Autodesk Inventor part; units mm, degrees
ref_plane "YZ Plane" through (0, 0, 0) normal (1, 0, 0) x (0, 1, 0)
ref_plane "XZ Plane" through (0, 0, 0) normal (0, 1, 0) x (-1, 0, 0)
ref_plane "XY Plane" through (0, 0, 0) normal (0, 0, 1) x (1, 0, 0)
ref_plane "Work Plane2" through (0, 5.2982, -18) normal (0, 0, -1) x (-1, 0, 0)
ref_plane "Work Plane4" through (0, -4.9464, -12) normal (0, 0, -1) x (-1, 0, 0)
ref_plane "Work Plane3" through (0, -4.9464, -7) normal (0, 0, -1) x (-1, 0, 0)
sketch "Sketch3" plane through (0, 5.2982, -18) normal (0, 0, -1) x (-1, 0, 0)
  line L0 (13, 53.6093) -> (-13, 53.6093)
  arc A0 (-13, 53.6093) -> (-30, 36.6093) centre (-13, 36.6093) ccw
  line L1 (-30, 36.6093) -> (-30, -44.3907)
  line L2 (-30, -44.3907) -> (30, -44.3907)
  line L3 (30, -44.3907) -> (30, 36.6093)
  arc A1 (30, 36.6093) -> (13, 53.6093) centre (13, 36.6093) ccw
  line L4 (-0.95, 23.6093) -> (-0.95, 40.6093)
  line L5 (-0.95, 40.6093) -> (0.95, 40.6093)
  line L6 (0.95, 40.6093) -> (0.95, 23.6093)
  line L7 (0.95, 23.6093) -> (-0.95, 23.6093)
  line L8 (6.55, 40.6093) -> (8.45, 40.6093)
  line L9 (8.45, 40.6093) -> (8.45, 23.6093)
  line L10 (8.45, 23.6093) -> (6.55, 23.6093)
  line L11 (6.55, 23.6093) -> (6.55, 40.6093)
  line L12 (-8.45, 40.6093) -> (-6.55, 40.6093)
  line L13 (-6.55, 40.6093) -> (-6.55, 23.6093)
  line L14 (-6.55, 23.6093) -> (-8.45, 23.6093)
  line L15 (-8.45, 23.6093) -> (-8.45, 40.6093)
  line L16 (-15.5, -21.0481) -> (-15.5, 10.5093)
  line L17 (-15.5, 10.5093) -> (-12, 10.5093)
  line L18 (-12, 10.5093) -> (-12, 4.9593)
  line L19 (-12, 4.9593) -> (12, 4.9593)
  line L20 (12, 4.9593) -> (12, 10.5093)
  line L21 (12, 10.5093) -> (15.5, 10.5093)
  line L22 (15.5, 10.5093) -> (15.5, -21.0481)
  arc A2 (17.5, -25.2907) -> (15.5, -21.0481) centre (12, -25.2907) ccw
  line L23 (17.5, -25.2907) -> (17.5, -34.7907)
  arc A3 (12, -40.2907) -> (17.5, -34.7907) centre (12, -34.7907) ccw
  line L24 (12, -40.2907) -> (-12, -40.2907)
  arc A4 (-17.5, -34.7907) -> (-12, -40.2907) centre (-12, -34.7907) ccw
  line L25 (-17.5, -34.7907) -> (-17.5, -25.2907)
  arc A5 (-15.5, -21.0481) -> (-17.5, -25.2907) centre (-12, -25.2907) ccw
  line L26 (-15.5, -0.3907) -> (15.5, -0.3907)
  line L27 (-15.5, -21.0481) -> (-15.5, -0.3907)
  arc A6 (-12, -19.7907) -> (-15.5, -21.0481) centre (-12, -25.2907) ccw
  line L28 (12, -19.7907) -> (-12, -19.7907)
  arc A7 (15.5, -21.0481) -> (12, -19.7907) centre (12, -25.2907) ccw
  line L29 (15.5, -0.3907) -> (15.5, -21.0481)
  arc A8 (-15, -21.2907) -> (-17, -25.2907) centre (-12, -25.2907) ccw
  line L30 (-17, -25.2907) -> (-17, -34.7907)
  arc A9 (-17, -34.7907) -> (-12, -39.7907) centre (-12, -34.7907) ccw
  line L31 (-12, -39.7907) -> (12, -39.7907)
  arc A10 (12, -39.7907) -> (17, -34.7907) centre (12, -34.7907) ccw
  line L32 (17, -34.7907) -> (17, -25.2907)
  arc A11 (17, -25.2907) -> (15, -21.2907) centre (12, -25.2907) ccw
  line L33 (-15, -21.2907) -> (-15, 10.0093)
  line L34 (-15, 10.0093) -> (-12.5, 10.0093)
  line L35 (-12.5, 10.0093) -> (-12.5, 4.4593)
  line L36 (-12.5, 4.4593) -> (12.5, 4.4593)
  line L37 (12.5, 4.4593) -> (12.5, 10.0093)
  line L38 (12.5, 10.0093) -> (15, 10.0093)
  line L39 (15, 10.0093) -> (15, -21.2907)
  point P0 (0, -5.2982)
  dimension "d3" = 0.5
  dimension "d4" = 0.5
extrude "Extrusion1" add sketch "Sketch3" against normal up to surface (5 mm away) from surface at -6 contours L33 L26 L39 A7 L28 A6 | A6 L28 A7 L39 A11 L32 A10 L31 A9 L30 A8 L33 | L33 L34 L35 L36 L37 L38 L39 L26
sketch "Sketch4" plane through (-12.5, 9.7575, -7) normal (0, 0, 1) x (1, 0, 0)
  line L0 (29.5, -39.25) -> (29.5, -29.75)
  arc A0 (29.5, -29.75) -> (27.5, -25.75) centre (24.5, -29.75) ccw
  line L1 (27.5, -25.75) -> (27.5, 5.55)
  line L2 (27.5, 5.55) -> (25, 5.55)
  line L3 (25, 5.55) -> (25, 0)
  line L4 (25, 0) -> (0, 0)
  line L5 (0, 0) -> (0, 5.55)
  line L6 (0, 5.55) -> (-2.5, 5.55)
  line L7 (-2.5, 5.55) -> (-2.5, -25.75)
  arc A1 (-2.5, -25.75) -> (-4.5, -29.75) centre (0.5, -29.75) ccw
  line L8 (-4.5, -29.75) -> (-4.5, -39.25)
  arc A2 (-4.5, -39.25) -> (0.5, -44.25) centre (0.5, -39.25) ccw
  line L9 (0.5, -44.25) -> (24.5, -44.25)
  arc A3 (24.5, -44.25) -> (29.5, -39.25) centre (24.5, -39.25) ccw
  line L10 (0.5, -24.25) -> (24.5, -24.25)
  arc A4 (0.5, -24.25) -> (-3, -25.5074) centre (0.5, -29.75) ccw
  arc A5 (28, -25.5074) -> (24.5, -24.25) centre (24.5, -29.75) ccw
  arc A6 (27.5, -25.75) -> (24.5, -24.75) centre (24.5, -29.75) ccw
  line L11 (24.5, -24.75) -> (0.5, -24.75)
  arc A7 (0.5, -24.75) -> (-2.5, -25.75) centre (0.5, -29.75) ccw
  point P0 (12.5, -9.7575)
extrude "Extrusion2" add sketch "Sketch4" along normal blind 6 contours A3 L9 A2 L8 A1 A7 L11 A6 A0 L0
sketch "Sketch5" plane through (0, 0, 0) normal (1, 0, 0) x (0, 1, 0)
  line L0 (9.7575, -7) -> (15.3075, -7)
  line L1 (4.9075, -6.5) -> (4.9075, -4)
  line L2 (15.8075, -4) -> (15.8075, -18)
  line L3 (15.3075, -7) -> (-15.9925, -7)
  line L4 (4.9075, -4) -> (15.8075, -4)
  line L5 (5.4075, -0.5) -> (5.4075, -7)
  line L6 (5.4075, -0.5) -> (15.3075, -4)
  line L7 (15.3075, -4) -> (15.3075, -7)
  point P0 (0, 0)
  dimension "d10" = 0.5
  dimension "d11" = 3.5
extrude "Extrusion3" add sketch "Sketch5" against normal up to surface (2.5 mm away) from surface at 15
mirror "Mirror1" about plane through (0, 0, 0) normal (1, 0, 0) of "Extrusion3"
sketch "Sketch6" plane through (0, 0, 0) normal (1, 0, 0) x (0, 1, 0)
  line L0 (5.4075, -7) -> (9.7575, -7)
  line L1 (5.4075, -0.5) -> (5.4075, -7)
  line L2 (5.4075, -0.5) -> (9.7575, -4)
  line L3 (9.7575, -4) -> (9.7575, -7)
  point P0 (0, 0)
  point P1 (15.3075, -4)
extrude "Extrusion4" add sketch "Sketch6" along normal up to surface (25 mm away) from surface at -12.5
properties part number "schnapper"
Geometry check sheet. Reference: the model listing, model coordinates, mm. A direction names the side the tool comes from. Round coordinates to 2 decimals unless told otherwise and drop trailing zeros. Loops run counter-clockwise (first coordinate to the right, second up) from the corner with the lowest first, then second, coordinate; pieces in that order, holes last. Notation, with made-up numbers: (42, -18.5) - (94, -18.5) arc R21 ccw to (94, -2.5) - close; hole circle Ø4 at (-26.75, -32.5). An arc over 180 degrees is marked (long way). One line per question, with ' | ' between items. Start each with the question number.
1. Cross-section at D-D on y = -9.5. Record the cut outline in (x, z), then the cut area to 3 significant figures.
2. Cross-section at B-B on x = 9. Record the cut outline in (y, z), then the cut area to 3 significant figures.
3. Cross-section at C-C on z = -10. Record the cut outline in (x, y).
4. Tool access check on faces 5 (the face through (0, 9.758, -8)), 6 (the face through (15, 3, -8)), 7 (the face through (-15, 3, -8)), 8 (the face through (0, -14.992, -4)), 9 (the face through (0, -25, -1)). Record the directions out of +Z, -Z, +X, -X, +Y, -Y that give a thin tool (end or side, any length) a straight path to the whole face; none if there is none.
5. Depth check by flat-ended pin: pin 1 (5 mm diameter, centred on y = 11, z = -8.5, fed in from -X); pin 2 (3 mm diameter, centred on x = 0, y = -28, fed in from +Z); pin 3 (2.5 mm diameter, centred on x = 0, z = -6.5, fed in from +Y). Enter the tip coordinate at first touch or a pass-through.
6. Cross-section at A-A on z = -5.25. Record the cut outline in (x, y).
7. Scan lines: line 1 (Y direction, x = -2, z = -6); line 2 (X direction, y = 8, z = -1.75); line 3 (Z direction, x = 9.5, y = -4). Record each from-to range of solid material in increasing order. Write a range as [from, to].
8. Draft check along Y on faces 1 (the face through (0, -5, -7)), 2 (the face through (-16.127, -17.17, -5.355)), 3 (the face through (-15.496, -33.067, -6.577)), 4 (the face through (17, -25, -7)). Enter one of: released by +Y, released by -Y, zero draft, split by the parting line, or undercut.
Taken from the geometry:
1) outline: (-15, -12) - (15, -12) - (15, -7) - (-15, -7) - close | area: 150 mm²
2) outline: (-34.49, -12) - (9.76, -12) - (9.76, -4) - (5.41, -0.5) - (5.41, -7) - (-14.99, -7) - (-14.99, -1) - (-34.49, -1) - close | area: 359 mm²
3) outline: (-17, -29.49) arc R5 ccw to (-12, -34.49) - (12, -34.49) arc R5 ccw to (17, -29.49) - (17, -19.99) arc R5 ccw to (15, -15.99) - (15, 15.31) - (12.5, 15.31) - (12.5, 9.76) - (-12.5, 9.76) - (-12.5, 15.31) - (-15, 15.31) - (-15, -15.99) arc R5 ccw to (-17, -19.99) - close
4) face 5: +Z, -Z, +Y | face 6: +Z, -Z, +X, +Y | face 7: +Z, -Z, -X, +Y | face 8: +Z, +X, -X | face 9: +Z, +X, -X, -Y
5) pin 1: x = -15 | pin 2: z = -1 | pin 3: y = 9.76
6) outline: (-17, -29.49) arc R5 ccw to (-12, -34.49) - (12, -34.49) arc R5 ccw to (17, -29.49) - (17, -19.99) arc R5 ccw to (12, -14.99) - (-12, -14.99) arc R5 ccw to (-17, -19.99) - close; (-15, 5.41) - (15, 5.41) - (15, 15.31) - (12.5, 15.31) - (12.5, 9.76) - (-12.5, 9.76) - (-12.5, 15.31) - (-15, 15.31) - close
7) line 1: [-34.49, -14.99], [5.41, 9.76] | line 2: [-15, -12.5], [12.5, 15] | line 3: [-12, -7]
8) face 1: undercut | face 2: undercut | face 3: released by -Y | face 4: zero draft
